Design review of the part built by this model. Coordinates are the model's own, in mm. A direction names the side the tool comes from. Give positions to 0.01 mm unless a question says otherwise; leave off trailing zeros. Order: outer loops, then holes, each group sorted by start corner. A loop starts at its lowest first (then second) coordinate and runs counter-clockwise, first axis right, second up. Notation, with made-up numbers: M -37.75,-13 L 7.25,-13 A31 ccw 7.25,12 Z; hole C 72,26 d9. An arc over 180 degrees is marked long. Answer as a JSON object with one key per item and string values.
Autodesk Inventor part; units mm, degrees
ref_plane "YZ Plane" through (0, 0, 0) normal (1, 0, 0) x (0, 1, 0)
ref_plane "XZ Plane" through (0, 0, 0) normal (0, 1, 0) x (-1, 0, 0)
ref_plane "XY Plane" through (0, 0, 0) normal (0, 0, 1) x (1, 0, 0)
sketch "Sketch1" plane through (0, 0, 0) normal (0, 0, 1) x (1, 0, 0)
  line L0 (-31.75, -6.35) -> (31.75, -6.35)
  line L1 (31.75, -6.35) -> (31.75, 6.35)
  line L2 (31.75, 6.35) -> (-31.75, 6.35)
  line L3 (-31.75, 6.35) -> (-31.75, -6.35)
  line L4 (-31.75, -6.35) -> (31.75, 6.35) construction
  line L5 (31.75, -6.35) -> (-31.75, 6.35) construction
  point P0 (0, 0)
  dimension "d0" = 63.5
  dimension "d1" = 12.7
extrude "Extrusion1" add sketch "Sketch1" along normal blind 158.75
sketch "Sketch2" plane through (-31.75, -6.35, 0) normal (0, -1, 0) x (1, 0, 0)
  line L0 (63.5, 0) -> (63.5, 158.75)
  line L1 (0, 95.25) -> (63.5, 95.25)
  line L2 (63.5, 95.25) -> (63.5, 158.75)
  line L3 (63.5, 158.75) -> (0, 158.75)
  line L4 (0, 158.75) -> (0, 95.25)
  line L5 (0, 95.25) -> (63.5, 158.75) construction
  line L6 (63.5, 95.25) -> (0, 158.75) construction
  point P0 (31.75, 0)
  point P1 (31.75, 127)
  dimension "d4" = 127
extrude "Extrusion2" cut sketch "Sketch2" against normal blind 6.35
sketch "Sketch3" plane through (0, 0, 0) normal (0, 0, -1) x (-1, 0, 0)
  line L0 (31.75, 0) -> (-31.75, 0)
  point P0 (0, 0)
  point P1 (-25.4, 0)
  point P2 (25.4, 0)
  dimension "d7" = 25.4
  dimension "d8" = 25.4
hole "Hole1" at (25.4, 0, 0) at (-25.4, 0, 0) direction (0, 0, 1) diameter 5.207 depth 12.7 tip angle 118
sketch "Sketch4" plane through (-31.75, 0, 0) normal (0, -1, 0) x (1, 0, 0)
  line L0 (0, 0) -> (63.5, 0)
  circle A0 centre (31.75, 127) radius 4.4323
  circle A1 centre (31.75, 127) radius 8.8646
  circle A2 centre (31.75, 127) radius 13.2969
  circle A3 centre (31.75, 127) radius 17.7292
  circle A4 centre (31.75, 127) radius 22.1615
  circle A5 centre (31.75, 127) radius 26.5938
  point P0 (31.75, 0)
  dimension "d16" = 127
  dimension "d17" = 8.8646
  dimension "d18" = 17.7292
  dimension "d19" = 26.5938
  dimension "d20" = 35.4584
  dimension "d21" = 44.323
  dimension "d33" = 53.1876
sketch "Sketch5" plane through (-31.75, 6.35, 0) normal (0, 1, 0) x (1, 0, 0)
  line L0 (63.5, 0) -> (0, 0)
  circle A0 centre (31.75, -127) radius 3.175
  point P0 (31.75, 0)
  dimension "d22" = 127
  dimension "d23" = 6.35
extrude "Extrusion3" cut sketch "Sketch5" against normal blind 5.842
hole "Hole2" at (0, 0, 127) direction (0, 1, 0) diameter 0.508 end through all
properties part number "target"
(1) We need section C-C (z = 143). Write out the cut boundary in (x, y).
Checked values:
{"outline": "M -31.75,0 L 31.75,0 L 31.75,6.35 L -31.75,6.35 Z"}
(2) Tool access review of faces 1 (the cylindrical face through (-0.41, 3.47, 123.85)), 2 (the cylindrical face through (-27.98, -0.34, 6.44)), 3 (the flat face through (-0.4, 0, 127.4)), 4 (the flat face through (0, 0, 0)), 5 (the flat face through (0, 6.35, 78)): name each direction out of +Z, -Z, +X, -X, +Y, -Y from which nothing blocks a thin tool from reaching the whole face with its end or side.
Checked values:
{"face 1": "+Y", "face 2": "-Z", "face 3": "+Z, +X, -X, -Y", "face 4": "-Z, +X, -X, +Y, -Y", "face 5": "+Z, -Z, +X, -X, +Y"}
(3) We need section A-A (x = 5). Write out the cut boundary in (y, z), plus the area to 3 significant figures.
Checked values:
{"outline": "M -6.35,0 L 6.35,0 L 6.35,158.75 L 0,158.75 L 0,95.25 L -6.35,95.25 Z", "area": "1,610 mm^2"}
(4) Draft analysis for pull direction X (two halves, no side actions). For faces 6 (the flat face through (0, -3, 95.25)), 7 (the flat face through (-31.75, 2, 61)), 8 (the flat face through (1, 0.508, 127)), state which applies: +X half, -X half, draft (parallel to the pull), parting line (faces both ways), or undercut.
Checked values:
{"face 6": "draft", "face 7": "-X half", "face 8": "undercut"}
(5) We need section B-B (y = -4.75). Write out the cut boundary in (x, z), plus the area to 3 significant figures.
Checked values:
{"outline": "M -31.75,0 L 31.75,0 L 31.75,95.25 L -31.75,95.25 Z", "area": "6,050 mm^2"}
(6) Insertion check: pin 1 (4 mm diameter, centred on x = -25.4, y = 0, fed in from -Z). The pin has a flat end and moves straight along its axis. Give the tip position at first contact, or say it passes through.
Checked values:
{"pin 1": "stops at z = 13.06"}
(7) To check wall thickness, follow L1, parallel to X at y = 0, z = 6.75; L2, parallel to X at y = 0.3, z = 127; L3, parallel to X at y = 3.15, z = 127 (3 decimals). State the ranges of each line that lie inside material, in increasing order. Write a range as from..to.
Checked values:
{"L1": "x = -31.75..-28, -22.8..22.8, 28..31.75", "L2": "x = -31.75..-0.25, 0.25..31.75", "L3": "x = -31.75..-3.175, 3.175..31.75"}
